Part model, mm, in its own coordinate system. A direction names the side the tool comes from. Round coordinates to 2 decimals unless told otherwise and drop trailing zeros. Loops run counter-clockwise (first coordinate to the right, second up) from the corner with the lowest first, then second, coordinate; pieces in that order, holes last. Notation, with made-up numbers: M 61.5,54 L 85.5,54 A12 cw 85.5,63 Z; hole C 43,31 d9. An arc over 180 degrees is marked long. Answer as CSV lines item,"result". Start each with the question number.
Item 1: Band-saw the part on A-A (z = 89). Give the cut face in (x, y), and give its area (3 significant figures).
Item 2: Band-saw the part on B-B (y = -2.5). Count the separate pieces of the cut face and the enclosed holes in it, and give its area (3 significant figures).
Item 3: Which spindle directions (+Z, -Z, +X, -X, +Y, -Y) get a long thin tool onto all of the face, cutting with end or side? Do faces 5 (the flat face through (21.636, -2, -2)), 6 (the flat face through (-12.68, -1.5, 30.92)). Say none if no direction does.
Item 4: Mould opens along X. For faces 1 (the cylindrical face through (-15.873, -1.503, 63.725)), 2 (the flat face through (25.691, -2, 0)), 3 (the flat face through (3, 0, 43)), 4 (the cylindrical face through (13.321, -1.503, 11.503)) say: pulls with the +X half, pulls with the -X half, needs draft (parallel to the pull), parting line crosses it, or undercut.
Item 5: Wall check: line 1 (Z direction, x = 43.5, y = -2); line 2 (X direction, y = -0.85, z = 65); line 3 (Z direction, x = -4, y = -1.15). Give the ranges that are in metal, low to high.
Item 6: Drop flat-ended pins along their axis: pin 1 Ø5.5 at (x, z) = (44.45, 0) entering from -Y; pin 2 Ø1.5 at (x, y) = (13.5, -1.5) entering from -Z; pin 3 Ø1 at (x, y) = (6, -0.5) entering from +Z; pin 4 Ø0.9 at (x, y) = (26.5, -1.5) entering from -Z. Give the stop position or say it passes through.
```python
from build123d import *

# Parameters (mm, degrees)
F0_R     = 3.175
F1_DEPTH = 3.048


with BuildPart() as f1:
    # F0 (on Front) → F1 (new body)
    with BuildSketch(Plane.XZ):
        with BuildLine():
            ThreePointArc((44.7334821429, -7.9324362036), (50.1620069047, -5.5115227815), (52.3875, 0))
            ThreePointArc((52.3875, 0), (50.1620069047, 5.5115227815), (44.7334821429, 7.9324362036))
            ThreePointArc((44.7334821429, 7.9324362036), (36.5125, 0), (44.7334821429, -7.9324362036))
        make_face()
        with Locations((44.45, 0)):
            Circle(F0_R, mode=Mode.SUBTRACT)
        with BuildLine():
            ThreePointArc((-9.4772553384, -0.9525), (-6.2623833816, -7.1769199091), (0.3401785714, -9.5189234444))
            ThreePointArc((0.3401785714, -9.5189234444), (6.8544082857, -6.6138273378), (9.525, 0))
            ThreePointArc((9.525, 0), (-0.4768479324, 9.5130563464), (-9.4772553384, -0.9525))
        make_face()
        Circle(F0_R, mode=Mode.SUBTRACT)
        with BuildLine():
            ThreePointArc((9.4502929642, 115.490625), (0, 123.825), (-9.4502929642, 115.490625))
            ThreePointArc((-9.4502929642, 115.490625), (-0.596483242, 104.7936951058), (9.525, 114.3))
            ThreePointArc((9.525, 114.3), (9.5063048942, 114.896483242), (9.4502929642, 115.490625))
        make_face()
        with Locations((0, 114.3)):
            Circle(F0_R, mode=Mode.SUBTRACT)
        with BuildLine():
            Line((-9.4502929642, 115.490625), (-15.7504882737, 65.484375))
            ThreePointArc((-15.7504882737, 65.484375), (0, 79.375), (15.7504882737, 65.484375))
            Line((15.7504882737, 65.484375), (9.4502929642, 115.490625))
            ThreePointArc((9.4502929642, 115.490625), (9.5063048942, 114.896483242), (9.525, 114.3))
            ThreePointArc((9.525, 114.3), (-0.596483242, 104.7936951058), (-9.4502929642, 115.490625))
        make_face()
        with Locations((-3.175, 100.0252)):
            Circle(F0_R, mode=Mode.SUBTRACT)
        with BuildLine():
            ThreePointArc((-15.7954255641, 61.9125), (0, 47.625), (15.7954255641, 61.9125))
            ThreePointArc((15.7954255641, 61.9125), (15.8550939106, 62.7052534459), (15.875, 63.5))
            ThreePointArc((15.875, 63.5), (15.8438414904, 64.4941387366), (15.7504882737, 65.484375))
            ThreePointArc((15.7504882737, 65.484375), (0, 79.375), (-15.7504882737, 65.484375))
            ThreePointArc((-15.7504882737, 65.484375), (-15.8737438155, 63.6997054867), (-15.7954255641, 61.9125))
        make_face()
        with Locations((0, 63.5)):
            Circle(F0_R, mode=Mode.SUBTRACT)
        with BuildLine():
            ThreePointArc((44.7334821429, -7.9324362036), (36.5125, 0), (44.7334821429, 7.9324362036))
            Line((44.7334821429, 7.9324362036), (18.9676000005, 8.8532337108))
            ThreePointArc((18.9676000005, 8.8532337108), (13.2611998974, 11.5713591498), (11.3411865923, 17.5933818124))
            Line((11.3411865923, 17.5933818124), (15.7954255641, 61.9125))
            ThreePointArc((15.7954255641, 61.9125), (0, 47.625), (-15.7954255641, 61.9125))
            Line((-15.7954255641, 61.9125), (-9.4772553384, -0.9525))
            ThreePointArc((-9.4772553384, -0.9525), (-0.4768479324, 9.5130563464), (9.525, 0))
            ThreePointArc((9.525, 0), (6.8544082857, -6.6138273378), (0.3401785714, -9.5189234444))
            Line((0.3401785714, -9.5189234444), (44.7334821429, -7.9324362036))
        make_face()
        with BuildLine():
            Line((18.1261931211, -4.8397090286), (17.1533066209, -4.8397090286))
            Line((17.1533066209, -4.8397090286), (13.6300027063, 4.3663431352))
            Line((13.6300027063, 4.3663431352), (13.5731752238, 4.3663431352))
            add(Edge.make_bspline(
                [(13.5731752238, 4.3663431352), (13.673191593, 3.272982372), (13.673191593, 1.7659175363)],
                knots=[0, 0, 0, 1, 1, 1], degree=2))
            Line((13.673191593, 1.7659175363), (13.673191593, -4.8397090286))
            Line((13.673191593, -4.8397090286), (12.5570998369, -4.8397090286))
            Line((12.5570998369, -4.8397090286), (12.5570998369, 5.5460816717))
            Line((12.5570998369, 5.5460816717), (14.3755792766, 5.5460816717))
            Line((14.3755792766, 5.5460816717), (17.6647539633, -3.0212295888))
            Line((17.6647539633, -3.0212295888), (17.7215814458, -3.0212295888))
            Line((17.7215814458, -3.0212295888), (21.0380333241, 5.5460816717))
            Line((21.0380333241, 5.5460816717), (22.842874168, 5.5460816717))
            Line((22.842874168, 5.5460816717), (22.842874168, -4.8397090286))
            Line((22.842874168, -4.8397090286), (21.6358584399, -4.8397090286))
            Line((21.6358584399, -4.8397090286), (21.6358584399, 1.8522953097))
            add(Edge.make_bspline(
                [(21.6358584399, 1.8522953097), (21.6358584399, 3.0024835554), (21.7358748091, 4.3527045394)],
                knots=[0, 0, 0, 1, 1, 1], degree=2))
            Line((21.7358748091, 4.3527045394), (21.6790473266, 4.3527045394))
            Line((21.6790473266, 4.3527045394), (18.1261931211, -4.8397090286))
        make_face(mode=Mode.SUBTRACT)
        with BuildLine():
            Line((25.6910675905, -4.8397090286), (25.6910675905, 5.5460816717))
            Line((25.6910675905, 5.5460816717), (28.6256387865, 5.5460816717))
            add(Edge.make_bspline(
                [(28.6256387865, 5.5460816717), (30.6918860499, 5.5460816717), (31.6159009152, 4.9277986622)],
                knots=[0, 0, 0, 1, 1, 1], degree=2))
            add(Edge.make_bspline(
                [(31.6159009152, 4.9277986622), (32.5399157805, 4.3095156527), (32.5399157805, 2.9752063638)],
                knots=[0, 0, 0, 1, 1, 1], degree=2))
            add(Edge.make_bspline(
                [(32.5399157805, 2.9752063638), (32.5399157805, 2.0500549488), (32.0250587892, 1.4499567337)],
                knots=[0, 0, 0, 1, 1, 1], degree=2))
            add(Edge.make_bspline(
                [(32.0250587892, 1.4499567337), (31.5102017978, 0.8498585186), (30.5214036024, 0.6725567732)],
                knots=[0, 0, 0, 1, 1, 1], degree=2))
            Line((30.5214036024, 0.6725567732), (30.5214036024, 0.6020906949))
            add(Edge.make_bspline(
                [(30.5214036024, 0.6020906949), (32.8876999734, 0.1974790195), (32.8876999734, -1.884679939)],
                knots=[0, 0, 0, 1, 1, 1], degree=2))
            add(Edge.make_bspline(
                [(32.8876999734, -1.884679939), (32.8876999734, -3.2758167104), (31.9466368633, -4.0577628695)],
                knots=[0, 0, 0, 1, 1, 1], degree=2))
            add(Edge.make_bspline(
                [(31.9466368633, -4.0577628695), (31.0055737532, -4.8397090286), (29.3143878743, -4.8397090286)],
                knots=[0, 0, 0, 1, 1, 1], degree=2))
            Line((29.3143878743, -4.8397090286), (25.6910675905, -4.8397090286))
        make_face(mode=Mode.SUBTRACT)
    extrude(amount=F1_DEPTH)


solid = f1.part
```
Answer block:
1,outline,"M -12.79,-3.05 L 12.79,-3.05 L 12.79,0 L -12.79,0 Z"
1,area,"78.0 mm^2"
2,separate pieces,"1"
2,enclosed holes,"7"
2,area,"3,660 mm^2"
3,face 5,"+Y, -Y"
3,face 6,"-Z, -X, +Y, -Y"
4,face 1,"pulls with the -X half"
4,face 2,"undercut"
4,face 3,"needs draft"
4,face 4,"pulls with the +X half"
5,line 1,"z = -7.98 to -3.03, 3.03 to 7.98"
5,line 2,"x = -15.8 to -2.8, 2.8 to 15.8"
5,line 3,"z = -8.64 to 96.96, 103.09 to 122.94"
6,pin 1,"passes through"
6,pin 2,"stops at z = -9.08"
6,pin 3,"stops at z = 122.08"
6,pin 4,"stops at z = -8.6"
